Read the model definition and answer for the solid it produces. Units are mm, in the model's axes. A direction names the side the tool comes from. Round coordinates to 2 decimals unless told otherwise and drop trailing zeros. Order: outer loops, then holes, each group sorted by start corner. A loop starts at its lowest first (then second) coordinate and runs counter-clockwise, first axis right, second up. Notation, with made-up numbers: (35, 10) - (75, 10) arc R19 cw to (75, 38) - close; hole circle Ø11 at (74, 66.25). An arc over 180 degrees is marked (long way). Answer as a JSON object with one key per item and string values. Group by question number.
Q1. A cutting plane is placed at B-B on y = 3. Determine the outline of the cut face in (x, z).
Q2. Consider line 1 (Y direction, x = 0, z = 0.75); line 2 (X direction, y = 3.25, z = 2); line 3 (Y direction, x = 1.25, z = -1). Determine where each line is inside the solid, lowest interval first.
Q3. A tool of negligible diameter and unlimited length cuts with its end or side. For faces 1 (the flat face through (0, -7.62, 0)), 2 (the cylindrical face through (-0.15, -3.76, -0.67)), from which of +Z, -Z, +X, -X, +Y, -Y can it reach the whole face along a straight path? Write none if from no direction.
Q4. Given pin 1 Ø2 at (x, y) = (0.5, 3.5) entering from -Z; pin 2 Ø1.5 at (x, z) = (-1.5, 0.5) entering from -Y; pin 3 Ø4 at (x, z) = (-2.5, 3) entering from +Y, each flat-ended and moving along its own axis, determine where each tip first touches the part or whether it passes through.
Q5. A cutting plane is placed at A-A on y = -5.75. Determine the outline of the cut face in (x, z), and give its area (3 significant figures).
```python
from build123d import *

# Parameters (mm, degrees)
SKETCH1_R           = 3.81
BOSS_EXTRUDE1_DEPTH = 6.35
SKETCH2_R           = 0.6858
BOSS_EXTRUDE2_DEPTH = 7.62
FILLET1_R           = 2.54


with BuildPart() as part:
    # Sketch1 → Boss-Extrude1 (new body)
    with BuildSketch(Plane(origin=(0, 0, 0), x_dir=(1, 0, 0), z_dir=(0, 1, 0))):
        Circle(SKETCH1_R)
    extrude(amount=BOSS_EXTRUDE1_DEPTH)

    # Sketch2 → Boss-Extrude2 (add)
    with BuildSketch(Plane.XZ):
        Circle(SKETCH2_R)
    extrude(amount=BOSS_EXTRUDE2_DEPTH)

    # Fillet1
    fillet1_edges = [part.edges().sort_by_distance(p)[0] for p in [
        (-3.81, 6.35, 0),
    ]]
    fillet(fillet1_edges, radius=FILLET1_R)


solid = part.part
```
Result set:
{
 "1": {"outline": "circle Ø7.62 at (0, 0)"},
 "2": {"line 1": "y = 0 to 6.35", "line 2": "x = -3.24 to 3.24", "line 3": "y = 0 to 6.33"},
 "3": {"face 1": "+Z, -Z, +X, -X, -Y", "face 2": "-Y"},
 "4": {"pin 1": "stops at z = -3.81", "pin 2": "stops at y = 0", "pin 3": "stops at y = 6.27"},
 "5": {"outline": "circle Ø1.37 at (0, 0)", "area": "1.48 mm²"}
}
